Input: dimensioned drawing with shaded views. Units: mm. Origin: part minimum x, y, z. Coordinates: 2 decimals unless noted, no trailing zeros. Order: outer loops, then holes, each group sorted by start corner. A loop starts at its lowest first (then second) coordinate and runs counter-clockwise, first axis right, second up. Notation, with made-up numbers: (67, 22) -> (125, 22) arc R28 cw to (125, 49) -> close; hole circle Ø7 at (-8.5, 28.25). An arc over 180 degrees is marked (long way). Answer as CSV lines item,"result".
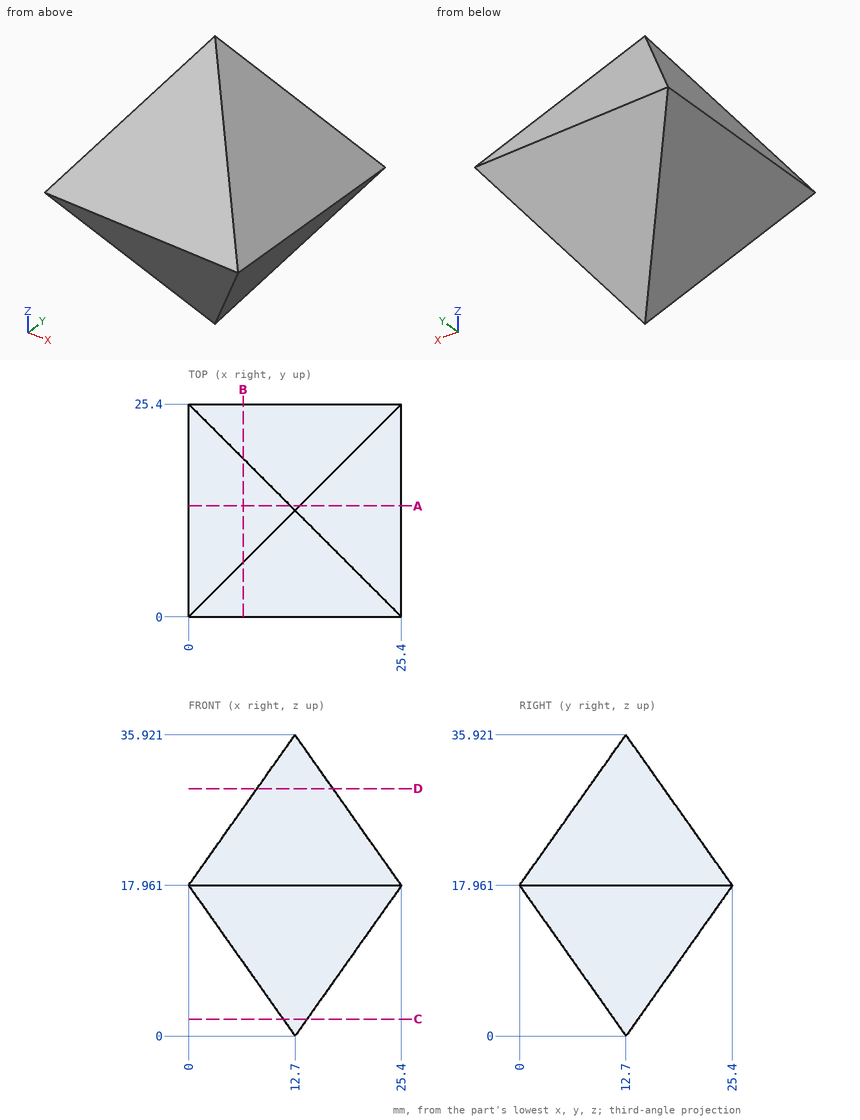
1. Cut plane B-B (x = 6.5). Return the cut outline in (y, z).
Findings:
outline,"(0, 17.96) -> (6.5, 8.77) -> (18.9, 8.77) -> (25.4, 17.96) -> (18.9, 27.15) -> (6.5, 27.15) -> close"
2. Contact query for flat-ended pins moving along their axis: pin 1 (5 mm diameter, centred on x = 2.5, y = 4, fed in from -Z); pin 2 (3 mm diameter, centred on x = 6, y = 6, fed in from +Z) (1 decimal); pin 3 (2 mm diameter, centred on y = 9.5, z = 19, fed in from -X); pin 4 (10 mm diameter, centred on x = 17, y = 13, fed in from +Z). Output: stop coordinate, or through.
Findings:
pin 1,"stops at z = 11.1"
pin 2,"stops at z = 27.9"
pin 3,"stops at x = 0.03"
pin 4,"stops at z = 35.92"
3. Cut plane D-D (z = 29.5). Return the cut outline in (x, y).
Findings:
outline,"(8.16, 8.16) -> (17.24, 8.16) -> (17.24, 17.24) -> (8.16, 17.24) -> close"
4. Cut plane A-A (y = 13.25). Return the cut outline in (x, z), plus the area to 3 significant figures.
Findings:
outline,"(0, 17.96) -> (12.15, 0.78) -> (13.25, 0.78) -> (25.4, 17.96) -> (13.25, 35.14) -> (12.15, 35.14) -> close"
area,"455 mm2"
5. Ray query, line 1 along Y through (x, z) = (9, 20); line 2 along Y through (x, z) = (22.25, 21); line 3 along Z through (x, y) = (10.25, 4.5) (1 decimal). Return the intervals inside material, ascending.
Findings:
line 1,"y = 1.44 to 23.96"
line 2,"y = 2.15 to 23.25"
line 3,"z = 11.6 to 24.3"
6. Cut plane C-C (z = 2). Return the cut outline in (x, y) (1 decimal).
Findings:
outline,"(11.3, 11.3) -> (14.1, 11.3) -> (14.1, 14.1) -> (11.3, 14.1) -> close"
